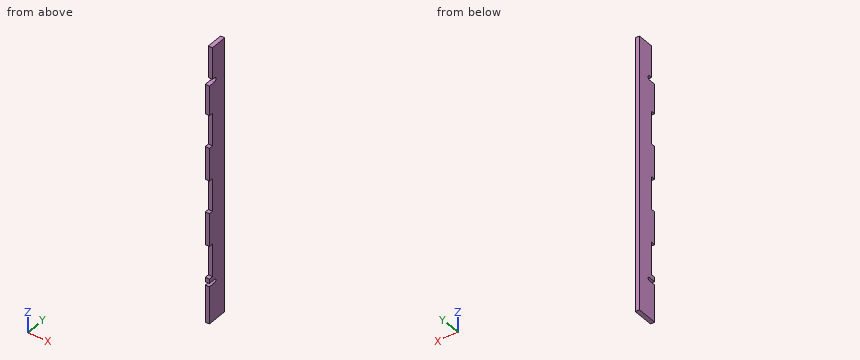
```python
from build123d import *

# Parameters (mm, degrees)
BOSS_EXTRUDE1_DEPTH = 6.35
CUT_EXTRUDE1_REACH  = 426.028
CUT_EXTRUDE2_DEPTH  = 425.027574582


with BuildPart() as part:
    # Sketch2 → Boss-Extrude1 (new body)
    with BuildSketch(Plane(origin=(0, 0, 0), x_dir=(0, 0, -1), z_dir=(1, 0, 0))):
        Polygon((48.319405744, 0), (99.119405744, 0), (99.119405744, 6.35), (149.919405744, 6.35), (149.919405744, 0), (200.719405744, 0), (200.719405744, 6.35), (251.519405744, 6.35), (251.519405744, 0), (302.319405744, 0), (302.319405744, 6.35), (353.119405744, 6.35), (353.119405744, 0), (422.789544579, 0), (422.789544579, 31.75), (-2.480594256, 31.75), (-2.480594256, 6.35), (48.319405744, 6.35), align=None)
    extrude(amount=BOSS_EXTRUDE1_DEPTH)

    # Sketch3 → Cut-Extrude1 (cut, up to next)
    with BuildSketch(Plane(origin=(6.35, 0, 0), x_dir=(0, 0, -1), z_dir=(1, 0, 0)), mode=Mode.PRIVATE) as cut_extrude1_sk1:
        with BuildLine():
            Line((365.019405744, 11.16), (365.019405744, -0.034586793))
            Line((365.019405744, -0.034586793), (360.019405744, -0.034586793))
            Line((360.019405744, -0.034586793), (360.019405744, 11.16))
            ThreePointArc((360.019405744, 11.16), (362.519405744, 13.66), (365.019405744, 11.16))
        make_face()
    cut_extrude1_tool1 = extrude(cut_extrude1_sk1.sketch, amount=-CUT_EXTRUDE1_REACH, mode=Mode.PRIVATE) & part.part
    add(cut_extrude1_tool1.solids().sort_by_distance((6.35, 6.556286, -362.519406))[0], mode=Mode.SUBTRACT)

    # Sketch4 → Cut-Extrude2 (cut, through all)
    with BuildSketch(Plane(origin=(6.35, 0, 0), x_dir=(0, 0, -1), z_dir=(1, 0, 0))):
        with BuildLine():
            Line((53.319405744, 10.31), (53.319405744, 0))
            Line((53.319405744, 0), (48.319405744, 0))
            Line((48.319405744, 0), (48.319405744, 6.35))
            Line((48.319405744, 6.35), (46.619405744, 6.35))
            Line((46.619405744, 6.35), (46.619405744, 10.31))
            ThreePointArc((46.619405744, 10.31), (49.969405744, 13.66), (53.319405744, 10.31))
        make_face()
    extrude(amount=-CUT_EXTRUDE2_DEPTH, mode=Mode.SUBTRACT)


solid = part.part
```
Design review of the part built by this model. Coordinates are the model's own, in mm. Give positions to 0.01 mm unless a question says otherwise; leave off trailing zeros. Write each loop counter-clockwise with the first axis right and the second up, starting at its lowest first coordinate (ties: lowest second). Pieces come first, ordered by that corner, then holes. Notation, with made-up numbers: (54.5, 29) - (59.5, 29) arc R11 ccw to (59.5, 40) - close; hole circle Ø2 at (81, -33.5). An arc over 180 degrees is marked (long way). Return JSON: item names as keys, results as strings. Group by question number.
(1) We need section B-B, the plane z = -339. Give the boundary of the cut face in (x, y), then the cut area to 3 significant figures.
(2) To check wall thickness, follow probe 1 along Z at (x, y) = (4.5, 3); probe 2 along Z at (x, y) = (4.25, 9.5); probe 3 along Z at (x, y) = (5.5, 12). State the ranges of each line that lie inside material, in increasing order.
(3) We need section A-A, the plane x = 5. Give the boundary of the cut face in (y, z), then the cut area to 3 significant figures.
(4) Insertion check: pin 1 (3 mm diameter, centred on x = 3.5, y = 3, fed in from +Z); pin 2 (3 mm diameter, centred on x = 4.5, z = -320, fed in from -Y); pin 3 (10 mm diameter, centred on y = 26.5, z = -213, fed in from -X). Each pin has a flat end and moves straight along its axis. Give the tip position at first contact, or say it passes through.
Reported:
{
 "1": {"outline": "(0, 6.35) - (6.35, 6.35) - (6.35, 31.75) - (0, 31.75) - close", "area": "161 mm2"},
 "2": {"probe 1": "z = -422.79 to -365.02, -360.02 to -353.12, -302.32 to -251.52, -200.72 to -149.92, -99.12 to -53.32", "probe 2": "z = -422.79 to -365.02, -360.02 to -53.32, -46.62 to 2.48", "probe 3": "z = -422.79 to -364.87, -360.16 to -52.86, -47.08 to 2.48"},
 "3": {"outline": "(0, -422.79) - (31.75, -422.79) - (31.75, 2.48) - (6.35, 2.48) - (6.35, -46.62) - (10.31, -46.62) arc R3.35 cw to (10.31, -53.32) - (0, -53.32) - (0, -99.12) - (6.35, -99.12) - (6.35, -149.92) - (0, -149.92) - (0, -200.72) - (6.35, -200.72) - (6.35, -251.52) - (0, -251.52) - (0, -302.32) - (6.35, -302.32) - (6.35, -353.12) - (0, -353.12) - (0, -360.02) - (11.16, -360.02) arc R2.5 cw to (11.16, -365.02) - (0, -365.02) - close", "area": "12,100 mm2"},
 "4": {"pin 1": "stops at z = -53.32", "pin 2": "stops at y = 6.35", "pin 3": "stops at x = 0"}
}
